For this review, use the dimensioned drawing (mm, ordinates from the lowest corner) and the shaded views. A direction names the side the tool comes from. Give positions to 0.01 mm unless a question says otherwise; leave off trailing zeros. Write each loop counter-clockwise with the first axis right and the second up, starting at its lowest first coordinate (ties: lowest second). Pieces come first, ordered by that corner, then holes. Notation, with made-up numbers: M 60,47 L 73,47 A26 ccw 73,83 Z; hole C 50,-20 d1. An arc over 180 degrees is marked long. One line per item, written item: value. Start each with the question number.
Item 1: Consider section A-A, the plane x = 17. Write out the cut boundary in (y, z).
Item 2: Consider section D-D, the plane y = 75. Write out the cut boundary in (x, z).
Item 3: Mouldability with a two-part tool opening along X and no side actions: class the marked faces 3, 4 and 5 as released by +X, released by -X, zero draft, split by the parting line, or undercut.
Item 4: Consider section B-B, the plane z = 12.5. Give the number of separate pieces and of enclosed holes in the cut face, and give its area (3 significant figures).
Item 5: Tool access review of the marked faces 1 and 2: name each direction out of +Z, -Z, +X, -X, +Y, -Y from which nothing blocks a thin tool from reaching the whole face with its end or side.
Item 6: Consider section C-C, the plane y = 20. Write out the cut boundary in (x, z), and give its area (3 significant figures).
Item 7: To check wall thickness, follow probe 1 along Y at (x, z) = (1, 12.5); probe 2 along X at (y, z) = (70, 21); probe 3 along Z at (x, y) = (23.9, 85). State the ranges of each line that lie inside material, in increasing order.
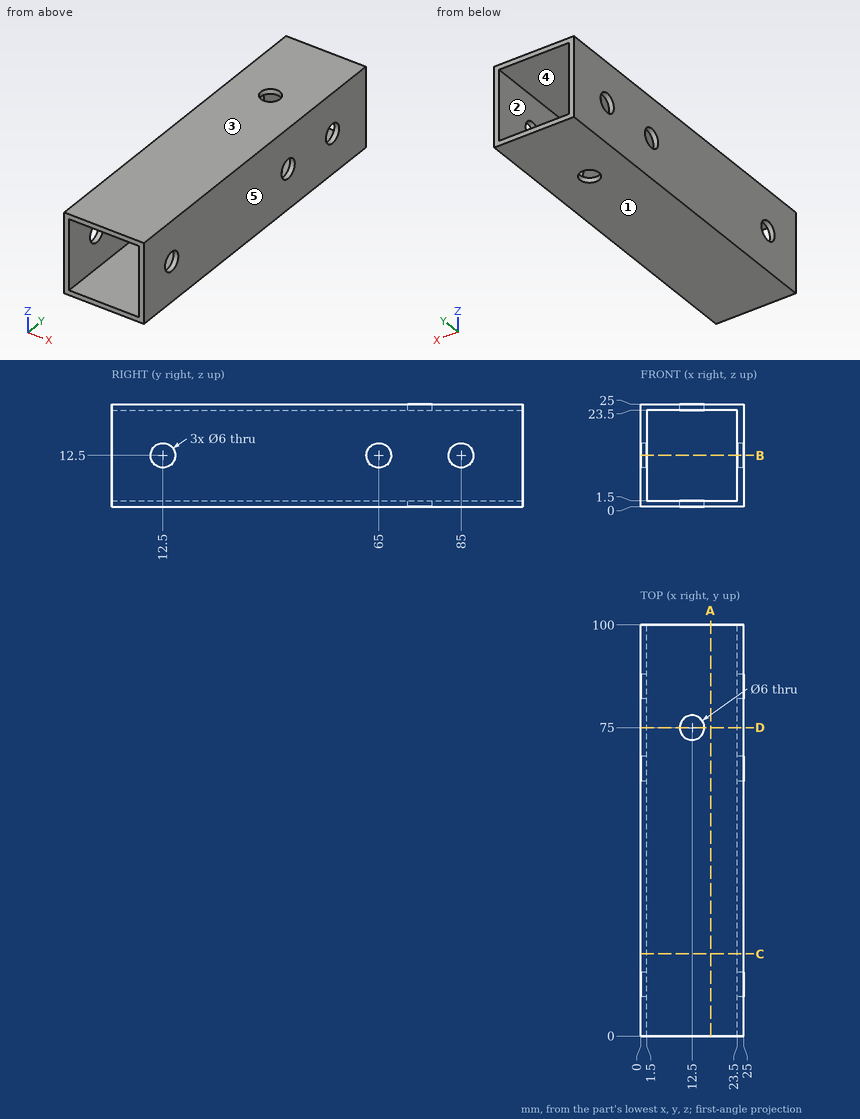
Model answer:
1. outline: M 0,0 L 100,0 L 100,1.5 L 0,1.5 Z; M 0,23.5 L 100,23.5 L 100,25 L 0,25 Z
2. outline: M 0,0 L 9.5,0 L 9.5,1.5 L 1.5,1.5 L 1.5,23.5 L 9.5,23.5 L 9.5,25 L 0,25 Z; M 15.5,0 L 25,0 L 25,25 L 15.5,25 L 15.5,23.5 L 23.5,23.5 L 23.5,1.5 L 15.5,1.5 Z
3. face 3: zero draft
3. face 4: undercut
3. face 5: released by +X
4. separate pieces: 8
4. enclosed holes: 0
4. area: 246 mm2
5. face 1: -Z, +X, -X, +Y, -Y
5. face 2: +Y, -Y
6. outline: M 0,0 L 25,0 L 25,25 L 0,25 Z; hole M 1.5,1.5 L 23.5,1.5 L 23.5,23.5 L 1.5,23.5 Z
6. area: 141 mm2
7. probe 1: y = 0 to 9.5, 15.5 to 62, 68 to 82, 88 to 100
7. probe 2: x = 0 to 1.5, 23.5 to 25
7. probe 3: z = 0 to 9.5, 15.5 to 25
